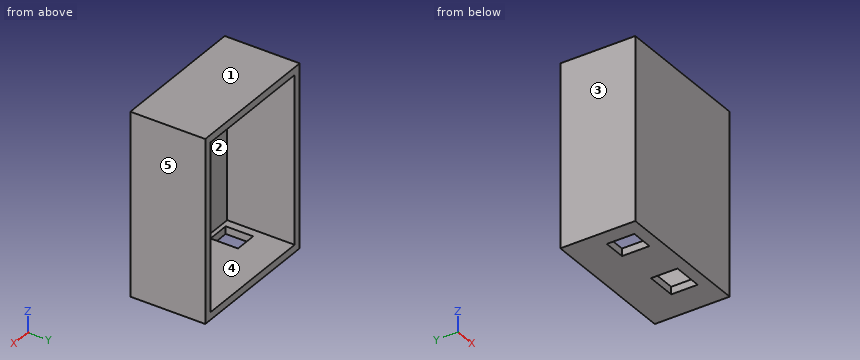
Autodesk Inventor part; units mm, degrees
ref_plane "YZ Plane" through (0, 0, 0) normal (1, 0, 0) x (0, 1, 0)
ref_plane "XZ Plane" through (0, 0, 0) normal (0, 1, 0) x (-1, 0, 0)
ref_plane "XY Plane" through (0, 0, 0) normal (0, 0, 1) x (1, 0, 0)
sketch "Sketch2" plane through (0, 0, 0) normal (0, 1, 0) x (-1, 0, 0)
  line L0 (0, 0) -> (-56, 0)
  line L1 (-56, 0) -> (-56, 73)
  line L2 (-56, 73) -> (0, 73)
  line L3 (0, 73) -> (0, 0)
  dimension "d0" = 56
  dimension "d1" = 73
extrude "Extrusion1" add sketch "Sketch2" along normal blind 30
shell "Shell1" thickness 3 removed faces 1 at (18.6667, 30, 24.3333)
sketch "Sketch3" plane through (56, 0, 0) normal (0, 0, -1) x (-1, 0, 0)
  line L0 (12, 15.3) -> (24, 15.3)
  line L1 (24, 15.3) -> (24, 4.7)
  line L2 (24, 4.7) -> (12, 4.7)
  line L3 (12, 4.7) -> (12, 15.3)
  line L4 (0, 0) -> (0, 30)
  line L5 (0, 0) -> (56, 0)
  line L6 (40.6, 15.7) -> (49.6, 15.7)
  line L7 (49.6, 15.7) -> (49.6, 4.7)
  line L8 (49.6, 4.7) -> (40.6, 4.7)
  line L9 (40.6, 4.7) -> (40.6, 15.7)
  line L10 (56, 0) -> (56, 30)
  dimension "d5" = 12
  dimension "d6" = 4.7
  dimension "d7" = 12
  dimension "d8" = 10.6
  dimension "d9" = 6.4
  dimension "d10" = 9
  dimension "d11" = 11
  dimension "d12" = 4.7
extrude "Extrusion2" cut sketch "Sketch3" against normal blind 30
equation "\"d12\" = d6"
properties part number "arduino array box v01"
Geometry check sheet. Reference: the model listing, model coordinates, mm. Face numbers are marked on the shaded views. A direction names the side the tool comes from. Give positions to 0.01 mm unless a question says otherwise; leave off trailing zeros. Write each loop counter-clockwise with the first axis right and the second up, starting at its lowest first coordinate (ties: lowest second). Pieces come first, ordered by that corner, then holes. Notation, with made-up numbers: (19, -5.75) -> (76, -5.75) arc R9 cw to (76, 11.25) -> close; hole circle Ø8 at (87.5, 28.5). An arc over 180 degrees is marked (long way). One line per question, with ' | ' between items.
Item 1: Draft check along X on the marked faces 1, 2 and 3. Enter one of: released by +X, released by -X, zero draft, split by the parting line, or undercut.
Determined:
face 1: zero draft | face 2: undercut | face 3: released by -X
Item 2: Sectioned sample at D-D, the plane y = 23. Record the boundary of the cut face in (x, z), plus the area to 3 significant figures.
Determined:
outline: (0, 0) -> (56, 0) -> (56, 73) -> (0, 73) -> close; hole (3, 3) -> (53, 3) -> (53, 70) -> (3, 70) -> close | area: 738 mm^2
Item 3: Access from +Z, -Z, +X, -X, +Y, -Y to the whole of each face (thin tool, end or side, straight path). Record for the marked faces 4 and 5.
Determined:
face 4: +Y | face 5: +Z, -Z, +X, +Y, -Y
Item 4: Sectioned sample at C-C, the plane x = 26. Record the boundary of the cut face in (y, z), plus the area to 3 significant figures.
Determined:
outline: (0, 0) -> (30, 0) -> (30, 3) -> (3, 3) -> (3, 70) -> (30, 70) -> (30, 73) -> (0, 73) -> close | area: 381 mm^2
Item 5: Depth check by flat-ended pin: pin 1 (0.9 mm diameter, centred on y = 8.5, z = 1.5, fed in from -X); pin 2 (15 mm diameter, centred on x = 26, z = 25.5, fed in from +Y). Enter the tip coordinate at first touch or a pass-through.
Determined:
pin 1: x = 0 | pin 2: y = 3
Item 6: Scan lines: line 1 along X through (y, z) = (20, 54.5); line 2 along Z through (x, y) = (28, 12.25); line 3 along Y through (x, z) = (36.5, 13.5). Record each from-to range of solid material in increasing order.
Determined:
line 1: 0 to 3, 53 to 56 | line 2: 0 to 3, 70 to 73 | line 3: 0 to 3
Item 7: Sectioned sample at B-B, the plane y = 12.5. Record the boundary of the cut face in (x, z).
Determined:
outline: (0, 0) -> (6.4, 0) -> (6.4, 3) -> (3, 3) -> (3, 70) -> (53, 70) -> (53, 3) -> (44, 3) -> (44, 0) -> (56, 0) -> (56, 73) -> (0, 73) -> close; (15.4, 0) -> (32, 0) -> (32, 3) -> (15.4, 3) -> close
Item 8: Sectioned sample at A-A, the plane x = 11. Record the boundary of the cut face in (y, z), plus the area to 3 significant figures.
Determined:
outline: (0, 0) -> (4.7, 0) -> (4.7, 3) -> (3, 3) -> (3, 70) -> (30, 70) -> (30, 73) -> (0, 73) -> close; (15.7, 0) -> (30, 0) -> (30, 3) -> (15.7, 3) -> close | area: 348 mm^2
